Model file for the job. Use its own axes, mm. Face numbers are marked on the shaded views. Coordinates: 2 decimals unless noted, no trailing zeros. Order: outer loops, then holes, each group sorted by start corner. A loop starts at its lowest first (then second) coordinate and runs counter-clockwise, first axis right, second up. Notation, with made-up numbers: (31.5, 78.5) -> (77.5, 78.5) arc R21 cw to (77.5, 89.5) -> close; hole circle Ø9 at (46, 19.5). An arc over 180 degrees is marked (long way). Use CSV: the item, a comma, the result in double quotes. Start each with the question number.
(1) Probe L1, parallel to Z at x = 0, y = -5.5; L2, parallel to Z at x = -2, y = -10.75; L3, parallel to Z at x = -16, y = -7.25. List the from-to ranges inside material, lowest first.
(2) Cut at B-B on y = -1.75. Write the cut outline in (x, z).
(3) Cut at D-D on x = -6. Write the cut outline in (y, z).
(4) Pin check, flat tips, straight feed: pin 1 Ø4 at (x, y) = (17, -2) entering from +Z; pin 2 Ø5 at (y, z) = (-2.5, 4.5) entering from -X; pin 3 Ø1 at (x, y) = (-7, -11.5) entering from +Z. Stop position of each tip, or through.
(5) Cut at A-A on x = 0. Write the cut outline in (y, z), plus the area to 3 significant figures.
(6) Cut at C-C on z = -2. Write the cut outline in (x, y).
(7) Pull direction Z, two halves, no side cores. Call the marked faces 1, 2, 3 and 4: pulls with the +Z half, pulls with the -Z half, needs draft (parallel to the pull), parting line crosses it, or undercut.
```python
from build123d import *

# Parameters (mm, degrees)
F0_R     = 2.54
F1_DEPTH = 12.7


with BuildPart() as f1:
    # F0 (on Front) → F1 (new body)
    with BuildSketch(Plane.XZ):
        with BuildLine():
            ThreePointArc((-23.876614939, 3.7876112691), (-20.9200976778, 2.836147849), (-19.6541820669, 0))
            Line((-19.6541820669, 0), (-6.35, 0))
            ThreePointArc((-6.35, 0), (-4.7269130816, 4.2401406485), (-0.6873881201, 6.3126854486))
            Line((-0.6873881201, 6.3126854486), (-23.876614939, 3.7876112691))
        make_face()
        with BuildLine():
            Line((-6.35, 0), (-19.6541820669, 0))
            ThreePointArc((-19.6541820669, 0), (-20.9200976778, -2.836147849), (-23.876614939, -3.7876112691))
            Line((-23.876614939, -3.7876112691), (-0.6873881201, -6.3126854486))
            ThreePointArc((-0.6873881201, -6.3126854486), (-4.7269130816, -4.2401406485), (-6.35, 0))
        make_face()
        with BuildLine():
            Line((24.1456229767, 3.7881261824), (0.6794606235, 6.3135436374))
            ThreePointArc((0.6794606235, 6.3135436374), (4.7242499383, 4.2431076489), (6.35, 0))
            Line((6.35, 0), (19.9279466026, 0))
            ThreePointArc((19.9279466026, 0), (21.1920820133, 2.834549963), (24.1456229767, 3.7881261824))
        make_face()
        with BuildLine():
            ThreePointArc((6.35, 0), (4.7242499383, -4.2431076489), (0.6794606235, -6.3135436374))
            Line((0.6794606235, -6.3135436374), (24.1456229767, -3.7881261824))
            ThreePointArc((24.1456229767, -3.7881261824), (21.1920820133, -2.834549963), (19.9279466026, 0))
            Line((19.9279466026, 0), (6.35, 0))
        make_face()
        with BuildLine():
            ThreePointArc((27.5479466026, 0), (26.5724965656, 2.5458645893), (24.1456229767, 3.7881261824))
            ThreePointArc((24.1456229767, 3.7881261824), (21.1920820133, 2.834549963), (19.9279466026, 0))
            ThreePointArc((19.9279466026, 0), (21.1920820133, -2.834549963), (24.1456229767, -3.7881261824))
            ThreePointArc((24.1456229767, -3.7881261824), (26.5724965656, -2.5458645893), (27.5479466026, 0))
        make_face()
        with BuildLine():
            ThreePointArc((26.2779466026, 0), (23.7379466026, -2.54), (21.1979466026, 0))
            ThreePointArc((21.1979466026, 0), (23.7379466026, 2.54), (26.2779466026, 0))
        make_face(mode=Mode.SUBTRACT)
        with BuildLine():
            ThreePointArc((-0.6873881201, 6.3126854486), (-4.7269130816, 4.2401406485), (-6.35, 0))
            Line((-6.35, 0), (-5.08, 0))
            ThreePointArc((-5.08, 0), (0, 5.08), (5.08, 0))
            Line((5.08, 0), (6.35, 0))
            ThreePointArc((6.35, 0), (4.7242499383, 4.2431076489), (0.6794606235, 6.3135436374))
            ThreePointArc((0.6794606235, 6.3135436374), (-0.0039869064, 6.3499987484), (-0.6873881201, 6.3126854486))
        make_face()
        with BuildLine():
            Line((-5.08, 0), (-6.35, 0))
            ThreePointArc((-6.35, 0), (-4.7269130816, -4.2401406485), (-0.6873881201, -6.3126854486))
            ThreePointArc((-0.6873881201, -6.3126854486), (-0.0039869064, -6.3499987484), (0.6794606235, -6.3135436374))
            ThreePointArc((0.6794606235, -6.3135436374), (4.7242499383, -4.2431076489), (6.35, 0))
            Line((6.35, 0), (5.08, 0))
            ThreePointArc((5.08, 0), (0, -5.08), (-5.08, 0))
        make_face()
        with BuildLine():
            ThreePointArc((-23.876614939, -3.7876112691), (-20.9200976778, -2.836147849), (-19.6541820669, 0))
            ThreePointArc((-19.6541820669, 0), (-20.9200976778, 2.836147849), (-23.876614939, 3.7876112691))
            ThreePointArc((-23.876614939, 3.7876112691), (-27.2741820669, 0), (-23.876614939, -3.7876112691))
        make_face()
        with Locations((-23.4641820669, 0)):
            Circle(F0_R, mode=Mode.SUBTRACT)
    extrude(amount=F1_DEPTH)


solid = f1.part
```
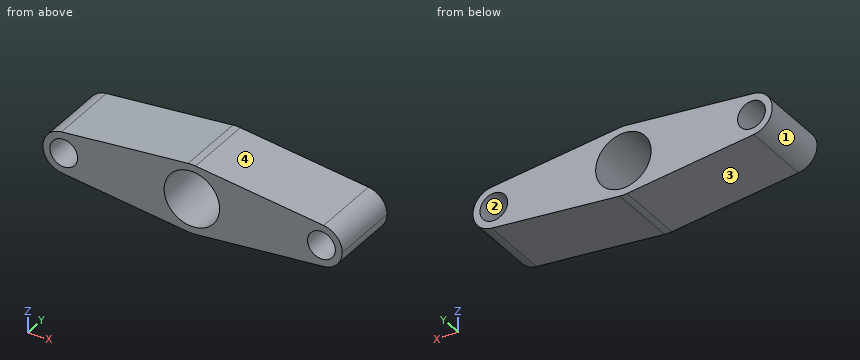
Outcome:
1,L1,"-6.35 to -5.08, 5.08 to 6.35"
1,L2,"-6.17 to -4.67, 4.67 to 6.17"
1,L3,"-4.65 to 4.65"
2,outline,"(-23.88, -3.79) -> (-0.69, -6.31) arc R6.35 ccw to (0.68, -6.31) -> (24.15, -3.79) arc R3.81 ccw to (24.15, 3.79) -> (0.68, 6.31) arc R6.35 ccw to (-0.69, 6.31) -> (-23.88, 3.79) arc R3.81 ccw to start; hole circle Ø5.08 at (-23.46, 0); hole circle Ø10.16 at (0, 0); hole circle Ø5.08 at (23.74, 0)"
3,outline,"(-12.7, -5.73) -> (0, -5.73) -> (0, 5.73) -> (-12.7, 5.73) -> close"
4,pin 1,"z = 4.77"
4,pin 2,"x = -26.71"
4,pin 3,"z = 5.68"
5,outline,"(-12.7, -6.35) -> (0, -6.35) -> (0, -5.08) -> (-12.7, -5.08) -> close; (-12.7, 5.08) -> (0, 5.08) -> (0, 6.35) -> (-12.7, 6.35) -> close"
5,area,"32.3 mm2"
6,outline,"(-26.71, -12.7) -> (-25.03, -12.7) -> (-25.03, 0) -> (-26.71, 0) -> close; (-21.9, -12.7) -> (-4.67, -12.7) -> (-4.67, 0) -> (-21.9, 0) -> close; (4.67, -12.7) -> (22.17, -12.7) -> (22.17, 0) -> (4.67, 0) -> close; (25.3, -12.7) -> (26.98, -12.7) -> (26.98, 0) -> (25.3, 0) -> close"
7,face 1,"parting line crosses it"
7,face 2,"undercut"
7,face 3,"pulls with the -Z half"
7,face 4,"pulls with the +Z half"
